Design review of the part built by this model. Coordinates are the model's own, in mm. A direction names the side the tool comes from. Coordinates: 2 decimals unless noted, no trailing zeros. Loops run counter-clockwise (first coordinate to the right, second up) from the corner with the lowest first, then second, coordinate; pieces in that order, holes last. Notation, with made-up numbers: M 61.5,16.25 L 91.5,16.25 A30 ccw 91.5,53.25 Z; hole C 63.5,-25.5 d10. An arc over 180 degrees is marked long. Put each result on its own line as item: value. Start each with the question number.
(1) Clearance check with flat-ended pins moving along their axes: pin 1 (3 mm diameter, centred on x = -20.5, z = 4, fed in from -Y); pin 2 (2 mm diameter, centred on x = 3, y = -0.5, fed in from +Z); pin 3 (3 mm diameter, centred on y = -4.5, z = -2, fed in from -X); pin 4 (8 mm diameter, centred on y = -1, z = 3, fed in from +X). State where each tip first meets the part, or that it passes through.
(2) For faces 4 (the flat face through (-4.445, 29.862, -6.338)), 5 (the flat face through (27.03, 13.46, -6.34)), 6 (the flat face through (-4.22, -13.23, 4.93)), 7 (the cylindrical face through (-2.38, -10.74, 6.55)), list the 3-axis set-ups (+Z, -Z, +X, -X, +Y, -Y) from which the entire face can be reached by the end or side of a thin tool; tool diameter is ignored.
(3) Take a section at B-B, the plane y = -8. Give the boundary of the cut face in (x, z), then the cut area to 3 significant figures.
(4) The part is to be moulded in two halves that separate along X. For faces 1 (the flat face through (22.289, 16.107, -5.07)), 2 (the cylindrical face through (24.3, -17.7, -12.5)), 3 (the flat face through (-19, 5.5, 5)), say which applies: +X half, -X half, draft (parallel to the pull), parting line (faces both ways), or undercut.
(5) Take a section at A-A, the plane z = -6.5. Give the boundary of the cut face in (x, y).
(6) For probe 1 along Y at (x, z) = (13, 5); probe 2 along X at (y, z) = (0.25, -4); probe 3 along Y at (x, z) = (-13, -8), list the stretches that pass through material, from the lowest coordinate up. Write a range as [from, to].
```python
from build123d import *
from build123d.topology import SkipClean

# Parameters (mm, degrees)
ESQUISSE1_R                  = 32.5
BOSS_EXTRU_1_DEPTH           = 10
ESQUISSE2_R                  = 1.5
BOSS_EXTRU_2_DEPTH           = 5
ENL_V_MAT_EXTRU_1_DEPTH      = 48.631397208
R_P_TITION_CIRCULAIRE1_COUNT = 5
ESQUISSE4_W                  = 11
ESQUISSE4_H                  = 11
ENL_V_MAT_EXTRU_3_DEPTH      = 48.631397303
R_P_TITION_CIRCULAIRE2_COUNT = 5
ESQUISSE5_R                  = 11
ENL_V_MAT_EXTRU_4_DEPTH      = 7


with BuildPart() as part:
    # Esquisse1 → Boss.-Extru.1 (new body)
    with BuildSketch(Plane.XY):
        Circle(ESQUISSE1_R)
    extrude(amount=BOSS_EXTRU_1_DEPTH)

    # Esquisse2 → Boss.-Extru.2 (add, symmetric)
    with BuildSketch(Plane(origin=(0, 0, 0), x_dir=(1, 0, 0), z_dir=(0, 1, 0))):
        with BuildLine():
            Line((-32.5, 0), (-32.5, 10))
            ThreePointArc((-32.5, 10), (-30, 12.5), (-27.5, 10))
            Line((-27.5, 10), (-27.5, 0))
            Line((-27.5, 0), (-32.5, 0))
        make_face()
        with Locations(Location((-30, 10, 0), (0, 0, 270))):
            Circle(ESQUISSE2_R, mode=Mode.SUBTRACT)
        with Locations(Location((-30, 4, 0), (0, 0, 270))):
            Circle(ESQUISSE2_R, mode=Mode.SUBTRACT)
    boss_extru_2 = extrude(amount=BOSS_EXTRU_2_DEPTH, both=True)

    # Esquisse3 → Enl_v. mat.-Extru.1 (cut, through all)
    with SkipClean():  # the faces are left unmerged after this step: merging them gives an invalid solid
        with BuildSketch(Plane.XY):
            with BuildLine():
                ThreePointArc((-32.5, 0), (-32.403125984, 2.507474126), (-32.113081447, 5))
                Line((-32.113081447, 5), (-32.5, 5))
                Line((-32.5, 5), (-32.5, 0))
            make_face()
            with BuildLine():
                ThreePointArc((-32.113081447, -5), (-32.403125984, -2.507474126), (-32.5, 0))
                Line((-32.5, 0), (-32.5, -5))
                Line((-32.5, -5), (-32.113081447, -5))
            make_face()
        enl_v_mat_extru_1 = extrude(amount=-ENL_V_MAT_EXTRU_1_DEPTH, mode=Mode.SUBTRACT)

    # R_p_tition circulaire1: Boss.-Extru.2, Enl_v. mat.-Extru.1 ×5 about axis
    with SkipClean():  # the faces are left unmerged after this step: merging them gives an invalid solid
        r_p_tition_circulaire1_axis = Axis((0, 0, 0), (0, 0, 1))
        add([boss_extru_2.rotate(r_p_tition_circulaire1_axis, i * 360 / R_P_TITION_CIRCULAIRE1_COUNT) for i in range(1, R_P_TITION_CIRCULAIRE1_COUNT)])
        add([enl_v_mat_extru_1.rotate(r_p_tition_circulaire1_axis, i * 360 / R_P_TITION_CIRCULAIRE1_COUNT) for i in range(1, R_P_TITION_CIRCULAIRE1_COUNT)], mode=Mode.SUBTRACT)

    # Esquisse4 → Enl_v. mat.-Extru.3 (cut, through all)
    with SkipClean():  # the faces are left unmerged after this step: merging them gives an invalid solid
        with BuildSketch(Plane(origin=(0, 0, 0), x_dir=(-1, 0, 0), z_dir=(0, 0, -1))):
            with Locations((19.386540723, 0)):
                Rectangle(ESQUISSE4_W, ESQUISSE4_H)
        enl_v_mat_extru_3 = extrude(amount=-ENL_V_MAT_EXTRU_3_DEPTH, mode=Mode.SUBTRACT)

    # R_p_tition circulaire2: Enl_v. mat.-Extru.3 ×5 about axis
    with SkipClean():  # the faces are left unmerged after this step: merging them gives an invalid solid
        r_p_tition_circulaire2_axis = Axis((0, 0, 0), (0, 0, 1))
        for i in range(1, R_P_TITION_CIRCULAIRE2_COUNT):
            add(enl_v_mat_extru_3.rotate(r_p_tition_circulaire2_axis, i * 360 / R_P_TITION_CIRCULAIRE2_COUNT), mode=Mode.SUBTRACT)

    # Esquisse5 → Enl_v. mat.-Extru.4 (cut)
    with SkipClean():  # the faces are left unmerged after this step: merging them gives an invalid solid
        with BuildSketch(Plane.XY.offset(10)):
            Circle(ESQUISSE5_R)
        extrude(amount=-ENL_V_MAT_EXTRU_4_DEPTH, mode=Mode.SUBTRACT)


solid = part.part
```
Computed values:
1. pin 1: stops at y = -26.37
1. pin 2: stops at z = 3
1. pin 3: stops at x = -32.36
1. pin 4: stops at x = 32.5
2. face 4: -Z, +X, +Y
2. face 5: -Z, +X
2. face 6: +Z, -Z
2. face 7: +Z
3. outline: M -31.5,0 L 11.35,0 L 11.35,10 L 7.55,10 L 7.55,3 L -7.55,3 L -7.55,10 L -31.5,10 Z; M 20.37,0 L 31.5,0 L 31.5,10 L 20.37,10 Z
3. area: 434 mm^2
4. face 1: -X half
4. face 2: parting line
4. face 3: undercut
5. outline: M -32.11,-5 L -27.5,-5 L -27.5,5 L -32.11,5 A32.5 ccw Z; M -14.68,-29 A32.5 ccw -5.17,-32.09 L -3.74,-27.7 L -13.25,-24.61 Z; M -14.68,29 L -13.25,24.61 L -3.74,27.7 L -5.17,32.09 A32.5 ccw Z; M 19.31,-20.21 L 23.04,-22.92 A32.5 ccw 28.92,-14.83 L 25.19,-12.12 Z; M 19.31,20.21 L 25.19,12.12 L 28.92,14.83 A32.5 ccw 23.04,22.92 Z
6. probe 1: y = [-29.79, -16.24], [-5.73, 5.73], [16.24, 29.79]
6. probe 2: x = [-32.5, -31.5], [-28.5, -27.5]
6. probe 3: y = [-29.79, -24.69], [24.69, 29.79]
